Check sheet for the drawn part. Datum: minimum x, y, z corner. Units: mm. A direction names the side the tool comes from. Give positions to 0.01 mm unless a question says otherwise; leave off trailing zeros. Write each loop counter-clockwise with the first axis right and the second up, starting at its lowest first coordinate (ties: lowest second). Pieces come first, ordered by that corner, then holes. Notation, with made-up numbers: M 69,85 L 127,85 A9 ccw 127,94 Z; hole C 51.5,75.5 d9. An arc over 180 degrees is marked long. Write item = value, one per line.
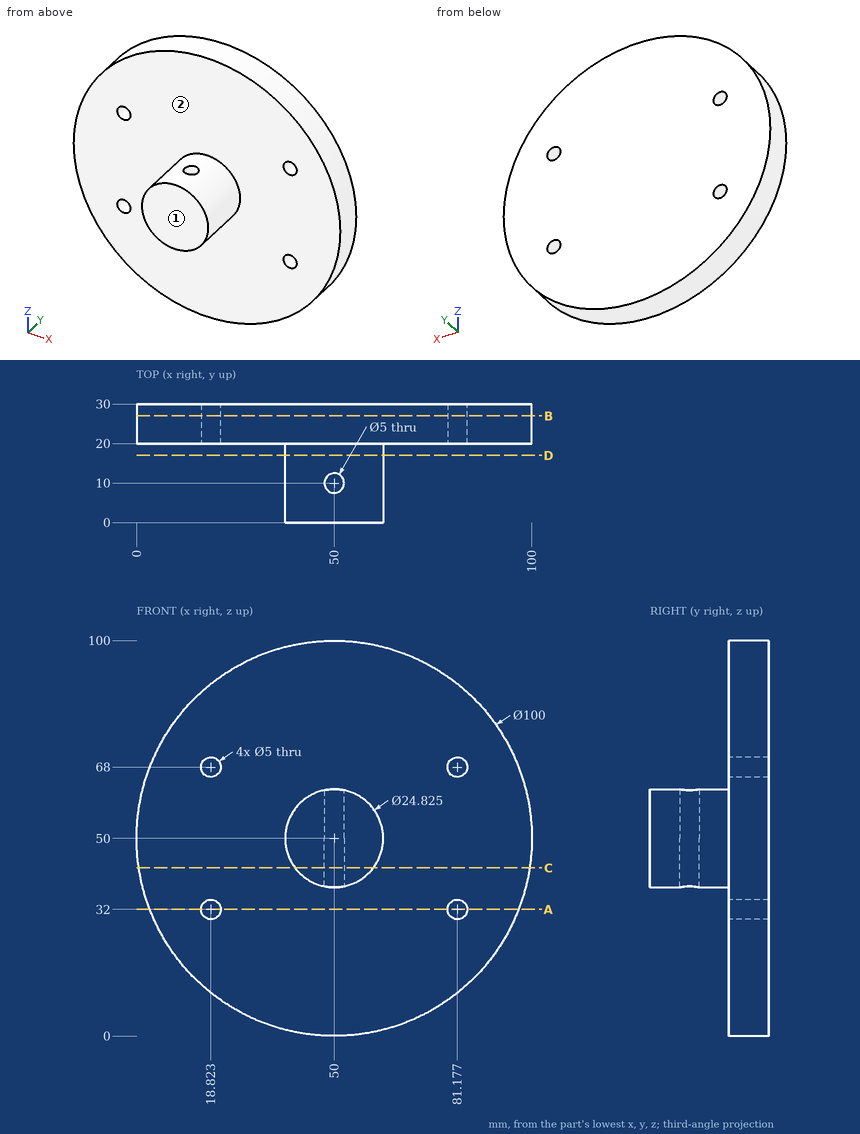
1) Cross-section at B-B on y = 27. Record the boundary of the cut face in (x, z), plus the area to 3 significant figures.
From the geometry:
outline = C 50,50 d100; hole C 18.82,32 d5; hole C 18.82,68 d5; hole C 81.18,32 d5; hole C 81.18,68 d5
area = 7,780 mm^2
2) Depth check by flat-ended pin: P1, Ø1.5, axis at y = 15.5, z = 46, coming from the +X side; P2, Ø3, axis at x = 81.18, z = 32, coming from the +Y side; P3, Ø1.5, axis at x = 21.5, y = 20.5, coming from the -Z side; P4, Ø4, axis at x = 50.5, y = 24.5, coming from the +Z side. Enter the tip coordinate at first touch or a pass-through.
From the geometry:
P1 = 61.98
P2 = through
P3 = 8.41
P4 = 100
3) Material ranges on probe 1 along Y at (x, z) = (50, 46); probe 2 along X at (y, z) = (26, 32); probe 3 along Y at (x, z) = (25, 19), recorded low to high. Write a range as from..to.
From the geometry:
probe_1 = 0..7.5, 12.5..30
probe_2 = 3.35..16.32, 21.32..78.68, 83.68..96.65
probe_3 = 20..30
4) Cross-section at A-A on z = 32. Record the boundary of the cut face in (x, y).
From the geometry:
outline = M 3.35,20 L 16.32,20 L 16.32,30 L 3.35,30 Z; M 21.32,20 L 78.68,20 L 78.68,30 L 21.32,30 Z; M 83.68,20 L 96.65,20 L 96.65,30 L 83.68,30 Z
5) Cross-section at D-D on y = 17. Record the boundary of the cut face in (x, z) (1 decimal), plus the area to 3 significant figures.
From the geometry:
outline = C 50,50 d24.8
area = 484 mm^2
6) Cross-section at C-C on z = 42.5. Record the boundary of the cut face in (x, y).
From the geometry:
outline = M 0.57,20 L 40.11,20 L 40.11,0 L 59.89,0 L 59.89,20 L 99.43,20 L 99.43,30 L 0.57,30 Z; hole C 50,10 d5
7) Tool access check on the marked faces 1 and 2. Record the directions out of +Z, -Z, +X, -X, +Y, -Y that give a thin tool (end or side, any length) a straight path to the whole face; none if there is none.
From the geometry:
face_1 = +Z, -Z, +X, -X, -Y
face_2 = -Y
